```python
from build123d import *

# Parameters (mm, degrees)
F1_DEPTH = 165
F2_R     = 10
F3_R     = 15
F5_DEPTH = 30


with BuildPart() as f1:
    # F0 (on Top) → F1 (new body)
    with BuildSketch(Plane.XY):
        with BuildLine():
            Line((-20, 60), (-100, 60))
            ThreePointArc((-100, 60), (-114.1421356237, 54.1421356237), (-120, 40))
            Line((-120, 40), (-120, -40))
            ThreePointArc((-120, -40), (-114.1421356237, -54.1421356237), (-100, -60))
            Line((-100, -60), (-20, -60))
            ThreePointArc((-20, -60), (-5.8578643763, -54.1421356237), (0, -40))
            Line((0, -40), (0, 40))
            ThreePointArc((0, 40), (-5.8578643763, 54.1421356237), (-20, 60))
        make_face()
    extrude(amount=F1_DEPTH)

    # F2
    f2_edges = [f1.edges().sort_by_distance(p)[0] for p in [
        (-60, -60, 0),
        (-114.142136, -54.142136, 0),
        (-5.857864, -54.142136, 0),
    ]]
    fillet(f2_edges, radius=F2_R)

    # F3
    f3_edges = [f1.edges().sort_by_distance(p)[0] for p in [
        (-60, 60, 165),
    ]]
    fillet(f3_edges, radius=F3_R)

    # F4 (on face) → F5 (join)
    with BuildSketch(Plane.XY.offset(165)):
        with BuildLine():
            Line((-15, -23.4956587879), (-15, 23.4956587879))
            ThreePointArc((-15, 23.4956587879), (-24.4613681652, 36.0235398418), (-37.3411373512, 45))
            Line((-37.3411373512, 45), (-80.9301267866, 45))
            ThreePointArc((-80.9301267866, 45), (-95.2159754206, 34.6151530926), (-105, 19.9112971522))
            Line((-105, 19.9112971522), (-105, -19.9112971522))
            ThreePointArc((-105, -19.9112971522), (-95.2159754206, -34.6151530926), (-80.9301267866, -45))
            Line((-80.9301267866, -45), (-37.3411373512, -45))
            ThreePointArc((-37.3411373512, -45), (-24.4613681652, -36.0235398418), (-15, -23.4956587879))
        make_face()
    extrude(amount=F5_DEPTH)


solid = f1.part
```
Model file for the job. Use its own axes, mm. A direction names the side the tool comes from. Round coordinates to 2 decimals unless told otherwise and drop trailing zeros. Loops run counter-clockwise (first coordinate to the right, second up) from the corner with the lowest first, then second, coordinate; pieces in that order, holes last. Notation, with made-up numbers: M 78.25,15 L 117.25,15 A20 cw 117.25,36 Z; hole C 34.25,-16 d8. An arc over 180 degrees is marked long. Put each result on its own line as item: value. Start each with the question number.
Item 1: Cut at C-C (x = -45.5). List the corners of the cut face in (y, z), then the cut area to 3 significant figures.
Item 2: 3-axis set-ups, long thin cutter, end or side, ignore diameter. For faces 1 (the face through (-95.043, 34.794, 179.79)), 2 (the face through (-105, 0, 180)), 3 (the face through (-24.3, 35.87, 179.79)), 4 (the face through (-59.44, -55.72, 160.49)), 5 (the face through (-15, 0, 180)): which of +Z, -Z, +X, -X, +Y, -Y reach the whole face in a straight line?
Item 3: Cut at D-D (y = -34). List the corners of the cut face in (x, z), then the cut area to 3 significant figures.
Item 4: Drill centre lines: line 1 along Y through (x, z) = (-100.5, 69); line 2 along Y through (x, z) = (-69.5, 184.5); line 3 along X through (y, z) = (5.5, 175). Where is each one in solid material? Low to high.
Item 5: Drop flat-ended pins along their axis: P1, Ø2, axis at y = 44.5, z = 45.5, coming from the +X side; P2, Ø15, axis at x = -70, z = 179, coming from the -Y side; P3, Ø24, axis at y = -1, z = 178, coming from the -X side. Give the stop position or say it passes through.
Item 6: Cut at A-A (z = 111.5). List the corners of the cut face in (x, y).
Item 7: Cut at B-B (y = -9). List the corners of the cut face in (x, z), then the cut area to 3 significant figures.
Answer block:
1. outline: M -60,10 A10 ccw -50,0 L 50,0 A10 ccw 60,10 L 60,150 A15 ccw 45,165 L 45,195 L -45,195 L -45,165 A15 ccw -60,150 Z
1. area: 22,400 mm2
2. face 1: +Z, -X, +Y
2. face 2: +Z, -X, +Y, -Y
2. face 3: +Z, +X, +Y
2. face 4: +Z, +X, -X, -Y
2. face 5: +Z, +X, +Y, -Y
3. outline: M -120,10 A10 ccw -110,0 L -10,0 A10 ccw 0,10 L 0,150 A15 ccw -15,165 L -22.48,165 L -22.48,195 L -95.8,195 L -95.8,165 L -105,165 A15 ccw -120,150 Z
3. area: 21,900 mm2
4. line 1: -59.99 to 59.99
4. line 2: -45 to 45
4. line 3: -105 to -15
5. P1: x = -0.31
5. P2: y = -45
5. P3: x = -105
6. outline: M -120,-40 A20 ccw -100,-60 L -20,-60 A20 ccw 0,-40 L 0,40 A20 ccw -20,60 L -100,60 A20 ccw -120,40 Z
7. outline: M -120,10 A10 ccw -110,0 L -10,0 A10 ccw 0,10 L 0,150 A15 ccw -15,165 L -15,195 L -105,195 L -105,165 A15 ccw -120,150 Z
7. area: 22,400 mm2
